Input: part model. Units: mm. Frame: model coordinates. Coordinates: 2 decimals unless noted, no trailing zeros. Write each loop counter-clockwise with the first axis right and the second up, starting at its lowest first coordinate (ties: lowest second). Pieces come first, ordered by that corner, then holes. Notation, with made-up numbers: M 84.5,-24.5 L 107.5,-24.5 A17 ccw 107.5,5.5 Z; hole C 75,61 d8. An arc over 180 degrees is marked long. Use CSV: the item, a comma, the result in double quotes.
```python
from build123d import *

# Parameters (mm, degrees)
BOSS_EXTRU_1_DEPTH       = 4
ESQUISSE2_W              = 130
ESQUISSE2_H              = 80
ENL_V_MAT_EXTRU_1_DEPTH  = 242.33172191
ESQUISSE3_W              = 3
ESQUISSE3_H              = 200
ENL_V_MAT_EXTRU_2_DEPTH  = 242.33172191
ESQUISSE4_R              = 2.1
ENL_V_MAT_EXTRU_3_DEPTH  = 242.33172191
ESQUISSE5_R              = 2
ENL_V_MAT_EXTRU_4_DEPTH  = 242.33172191
ESQUISSE7_R              = 3.25
ENL_V_MAT_EXTRU_6_DEPTH  = 242.33172191
ESQUISSE8_W              = 5.4
ESQUISSE8_H              = 30.4
ENL_V_MAT_EXTRU_7_DEPTH  = 242.33172191
ESQUISSE9_W              = 4.4
ESQUISSE9_H              = 10.4
ENL_V_MAT_EXTRU_8_DEPTH  = 4.2
ENL_V_MAT_EXTRU_9_DEPTH  = 242.33172191
ESQUISSE12_W             = 14.6
ESQUISSE12_H             = 4
BOSS_EXTRU_2_DEPTH       = 4
ENL_V_MAT_EXTRU_10_DEPTH = 242.33172191
ENL_V_MAT_EXTRU_11_DEPTH = 242.33172191
ENL_V_MAT_EXTRU_12_DEPTH = 242.33172191
ESQUISSE16_R             = 2.1
ENL_V_MAT_EXTRU_13_DEPTH = 242.33172191


with BuildPart() as part:
    # Esquisse1 → Boss.-Extru.1 (new body)
    with BuildSketch(Plane.XY):
        Polygon((0, 0), (-135, 0), (-135, 200), (111, 200), (111, -80), (35, -80), align=None)
    extrude(amount=BOSS_EXTRU_1_DEPTH)

    # Esquisse2 → Enlèv. mat.-Extru.1 (cut, through all)
    with BuildSketch(Plane.XY.offset(4)):
        with Locations((-70, 140)):
            Rectangle(ESQUISSE2_W, ESQUISSE2_H)
    extrude(amount=-ENL_V_MAT_EXTRU_1_DEPTH, mode=Mode.SUBTRACT)

    # Esquisse3 → Enlèv. mat.-Extru.2 (cut, through all)
    with BuildSketch(Plane.XY.offset(4)):
        with Locations((109.5, 40)):
            Rectangle(ESQUISSE3_W, ESQUISSE3_H)
    extrude(amount=-ENL_V_MAT_EXTRU_2_DEPTH, mode=Mode.SUBTRACT)

    # Esquisse4 → Enlèv. mat.-Extru.3 (cut, through all)
    with BuildSketch(Plane.XY.offset(4)):
        with Locations((24.132044328, 83.658479689)):
            Circle(ESQUISSE4_R)
        with Locations((87.332280645, 53.563129062)):
            Circle(ESQUISSE4_R)
        with Locations((2.5, 110)):
            Circle(ESQUISSE4_R)
        with Locations((2.5, 180)):
            Circle(ESQUISSE4_R)
    extrude(amount=-ENL_V_MAT_EXTRU_3_DEPTH, mode=Mode.SUBTRACT)

    # Esquisse5 → Enlèv. mat.-Extru.4 (cut, through all)
    with BuildSketch(Plane.XY.offset(4)):
        with Locations((-110, 30)):
            Circle(ESQUISSE5_R)
    extrude(amount=-ENL_V_MAT_EXTRU_4_DEPTH, mode=Mode.SUBTRACT)

    # Esquisse7 → Enlèv. mat.-Extru.6 (cut, through all)
    with BuildSketch(Plane(origin=(0, 0, 0), x_dir=(-1, 0, 0), z_dir=(0, 0, -1))):
        with Locations((-20, 185)):
            Circle(ESQUISSE7_R)
    extrude(amount=-ENL_V_MAT_EXTRU_6_DEPTH, mode=Mode.SUBTRACT)

    # Esquisse8 → Enlèv. mat.-Extru.7 (cut, through all)
    with BuildSketch(Plane.XY.offset(4)):
        with Locations((2.5, 145)):
            Rectangle(ESQUISSE8_W, ESQUISSE8_H)
        Polygon((68.294821705, 59.638090553), (70.616463039, 64.513537354), (43.169503267, 77.583518198), (40.847861933, 72.708071397), align=None)
    extrude(amount=-ENL_V_MAT_EXTRU_7_DEPTH, mode=Mode.SUBTRACT)

    # Esquisse9 → Enlèv. mat.-Extru.8 (cut)
    with BuildSketch(Plane.ZY.offset(135)):
        with Locations((2, 95)):
            Rectangle(ESQUISSE9_W, ESQUISSE9_H)
        with Locations((2, 55.385186032)):
            Rectangle(ESQUISSE9_W, ESQUISSE9_H)
        with Locations((2, 75.192593016)):
            Rectangle(ESQUISSE9_W, ESQUISSE9_H)
    extrude(amount=-ENL_V_MAT_EXTRU_8_DEPTH, mode=Mode.SUBTRACT)

    # Esquisse10 → Enlèv. mat.-Extru.9 (cut, through all)
    with BuildSketch(Plane.XY.offset(4)):
        Polygon((-130.8, 77.292593016), (-124, 77.292593016), (-124, 78.692593016), (-120.8, 78.692593016), (-120.8, 77.292593016), (-113.8, 77.292593016), (-113.8, 73.092593016), (-120.8, 73.092593016), (-120.8, 71.692593016), (-124, 71.692593016), (-124, 73.092593016), (-130.8, 73.092593016), align=None)
    extrude(amount=-ENL_V_MAT_EXTRU_9_DEPTH, mode=Mode.SUBTRACT)

    # Esquisse12 → Boss.-Extru.2 (add)
    with BuildSketch(Plane(origin=(0, 0, 0), x_dir=(-1, 0, 0), z_dir=(0, 0, -1))):
        with Locations((-42.5, -82)):
            Rectangle(ESQUISSE12_W, ESQUISSE12_H)
        with Locations((-102.5, -82)):
            Rectangle(ESQUISSE12_W, ESQUISSE12_H)
        with BuildLine():
            Line((-67.5, -82), (-67.5, -80))
            Line((-67.5, -80), (-77.5, -80))
            Line((-77.5, -80), (-77.5, -82))
            ThreePointArc((-77.5, -82), (-72.5, -87), (-67.5, -82))
        make_face()
    extrude(amount=-BOSS_EXTRU_2_DEPTH)

    # Esquisse13 → Enlèv. mat.-Extru.10 (cut, through all)
    with BuildSketch(Plane(origin=(0, 0, 0), x_dir=(-1, 0, 0), z_dir=(0, 0, -1))):
        Polygon((-18.341719551, -41.923930403), (-16.658280449, -38.076069597), (-22.888150326, -35.350501525), (-22.327003958, -34.067881257), (-25.25870743, -32.785260988), (-25.819853798, -34.067881257), (-32.232955142, -31.262149418), (-33.916394245, -35.110010225), (-27.5032929, -37.915742063), (-28.064439268, -39.198362332), (-25.132735796, -40.480982601), (-24.571589429, -39.198362332), align=None)
    extrude(amount=-ENL_V_MAT_EXTRU_10_DEPTH, mode=Mode.SUBTRACT)

    # Esquisse14 → Enlèv. mat.-Extru.11 (cut, through all)
    with BuildSketch(Plane(origin=(0, 0, 0), x_dir=(-1, 0, 0), z_dir=(0, 0, -1))):
        Polygon((-104.2, 172.1), (-104.2, 173.5), (-101, 173.5), (-101, 172.1), (-94, 172.1), (-94, 167.9), (-101, 167.9), (-101, 166.5), (-104.2, 166.5), (-104.2, 167.9), (-111, 167.9), (-111, 172.1), align=None)
    extrude(amount=-ENL_V_MAT_EXTRU_11_DEPTH, mode=Mode.SUBTRACT)

    # Esquisse15 → Enlèv. mat.-Extru.12 (cut, through all)
    with BuildSketch(Plane.XY.offset(4)):
        Polygon((-69.6, 17), (-65.4, 17), (-65.4, 9), (-64, 9), (-64, 5.8), (-65.4, 5.8), (-65.4, 0), (-69.6, 0), (-69.6, 5.8), (-71, 5.8), (-71, 9), (-69.6, 9), align=None)
    extrude(amount=-ENL_V_MAT_EXTRU_12_DEPTH, mode=Mode.SUBTRACT)

    # Esquisse16 → Enlèv. mat.-Extru.13 (cut, through all)
    with BuildSketch(Plane.XY.offset(4)):
        with Locations((72.5, -82)):
            Circle(ESQUISSE16_R)
    extrude(amount=-ENL_V_MAT_EXTRU_13_DEPTH, mode=Mode.SUBTRACT)


solid = part.part
```
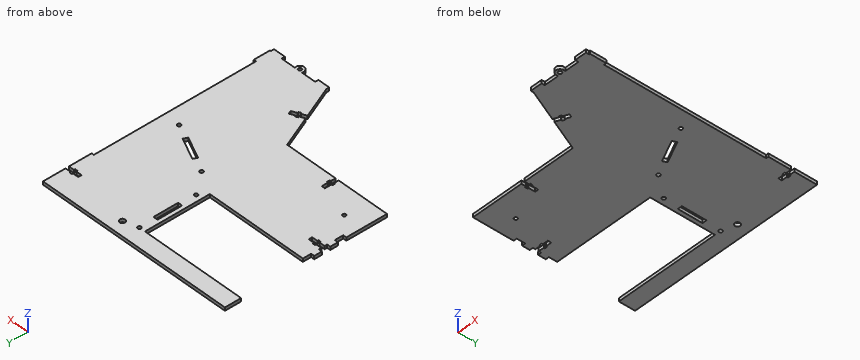
1. Section C-C (y = -66.5). Return loops of the section in (x, z), then the cut area to 3 significant figures.
Resolved:
outline,"M 29.09,0 L 111,0 L 111,4 L 29.09,4 Z"
area,"328 mm^2"
2. Section B-B (z = 2.6). State how many separate pieces and enclosed holes the cut face has, then the cut area to 3 significant figures.
Resolved:
separate pieces,"1"
enclosed holes,"9"
area,"45,000 mm^2"
3. Section A-A (x = -25). Return loops of the section in (y, z), then the cut area to 3 significant figures.
Resolved:
outline,"M 0,0 L 100,0 L 100,4 L 0,4 Z; M 180,0 L 200,0 L 200,4 L 180,4 Z"
area,"480 mm^2"
4. Contact query for flat-ended pins moving along their axis: pin 1 Ø1.5 at (x, z) = (-107.5, 2.5) entering from -Y; pin 2 Ø1.1 at (y, z) = (172.5, 1.5) entering from -X; pin 3 Ø1 at (x, z) = (102.5, 2) entering from -Y. Output: stop coordinate, or through.
Resolved:
pin 1,"stops at y = 0"
pin 2,"stops at x = -5"
pin 3,"stops at y = -84"
5. Material intervals for line 1 (Y direction, x = -114, z = 2.8); line 2 (Y direction, x = -110, z = 1.1); line 3 (Y direction, x = -54.5, z = 1.6), sorted ascending. Write a range as [from, to].
Resolved:
line 1,"y = [0, 73.09], [77.29, 100], [180, 200]"
line 2,"y = [0, 28], [32, 100], [180, 200]"
line 3,"y = [0, 100], [180, 200]"
